Geometry: final body of the model. Coordinates: model frame, mm. Face numbers are marked on the shaded views. A direction names the side the tool comes from. Coordinates: 2 decimals unless noted, no trailing zeros. Loops run counter-clockwise (first coordinate to the right, second up) from the corner with the lowest first, then second, coordinate; pieces in that order, holes last. Notation, with made-up numbers: (42.5, -10.5) - (70.5, -10.5) arc R28 cw to (70.5, 9.5) - close; hole circle Ø6 at (-26, 83.25). An arc over 180 degrees is marked (long way). Put each result on its own line as item: value. Start each with the question number.
1) Section D-D on y = 1.5. Output: boundary loops of the cut face in (x, z).
2) Section B-B on z = -1.4. Output: boundary loops of the cut face in (x, y), and give its area (3 significant figures).
3) Section A-A on x = 2.75. Output: boundary loops of the cut face in (y, z).
4) Reachability of the marked faces 1, 2, 3 and 4 from +Z, -Z, +X, -X, +Y, -Y: full face, straight path, thin tool, end or side. Return the list, or none.
5) Section C-C on y = 17. Output: boundary loops of the cut face in (x, z).
6) Draft query along X for the marked faces 5, 6 and 7. Return one class per face: +X half, -X half, draft (parallel to the pull), parting line (faces both ways), or undercut.
7) Material intervals for line 1 along X through (y, z) = (15.5, -2.8); line 2 along X through (y, z) = (13.5, -1.95); line 3 along Y through (x, z) = (3.5, -2.05), sorted ascending. Write a range as from..to.
8) Contact query for a flat-ended pin moving along its axis: pin 1 Ø8 at (x, y) = (0.5, 5.5) entering from +Z. Output: stop coordinate, or through.
```python
from build123d import *

# Parameters (mm, degrees)
SKETCH_1_R      = 1.3
EXTRUDE_1_DEPTH = 3


with BuildPart() as part:
    # 草图1 → 凸台-拉伸1 (new body)
    with BuildSketch(Plane(origin=(0, 0, -3.362857667), x_dir=(-1, 0, 0), z_dir=(0, 0, -1))):
        with BuildLine():
            Line((-8.929456987, 17.45330102), (-12.208534908, 5.216337034))
            ThreePointArc((-12.208534908, 5.216337034), (-8.203956956, -0.691485495), (-5.819308033, 6.03550946))
            ThreePointArc((-5.819308033, 6.03550946), (-6.310108859, 6.921233679), (-6.304159928, 7.933833034))
            Line((-6.304159928, 7.933833034), (-4.539684391, 14.518557193))
            ThreePointArc((-4.539684391, 14.518557193), (-3.62301138, 15.532716808), (-2.264294404, 15.382060533))
            Line((-2.264294404, 15.382060533), (-0.142530428, 17.503217343))
            Line((-0.142530428, 17.503217343), (4.099819599, 13.25965297))
            Line((4.099819599, 13.25965297), (5.797509256, 14.956856814))
            Line((5.797509256, 14.956856814), (1.554532399, 19.201048196))
            Line((1.554532399, 19.201048196), (3.675778765, 21.321687543))
            Line((3.675778765, 21.321687543), (-4.808443123, 29.808337985))
            Line((-4.808443123, 29.808337985), (-6.931968366, 27.685420414))
            Line((-6.931968366, 27.685420414), (-11.173246227, 31.927912314))
            Line((-11.173246227, 31.927912314), (-12.870428791, 30.231215419))
            Line((-12.870428791, 30.231215419), (-8.629080401, 25.98865297))
            Line((-8.629080401, 25.98865297), (-10.749072595, 23.869267436))
            Line((-10.749072595, 23.869267436), (-10.611098311, 23.731253658))
            ThreePointArc((-10.611098311, 23.731253658), (-8.929299443, 20.817545637), (-8.929456987, 17.45330102))
        make_face()
        with Locations(Location((-3.536567574, 22.593983824, 0), (0, 0, 180))):
            Circle(SKETCH_1_R, mode=Mode.SUBTRACT)
        with Locations(Location((-8.71249984, 3.274951558, 0), (0, 0, 180))):
            Circle(SKETCH_1_R, mode=Mode.SUBTRACT)
    extrude(amount=-EXTRUDE_1_DEPTH)


solid = part.part
```
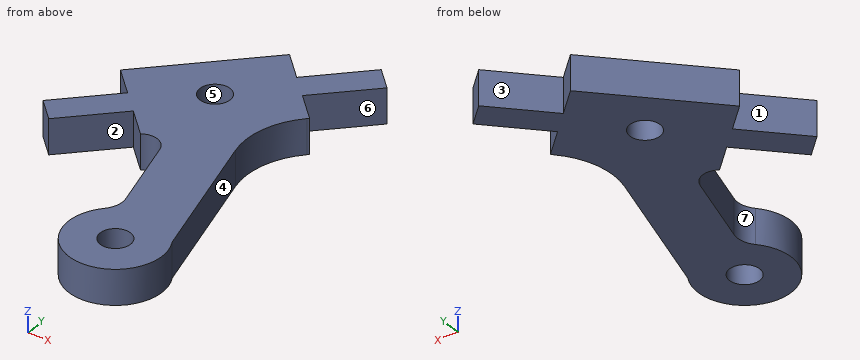
Answer block:
1. outline: (5.13, -3.36) - (12.3, -3.36) - (12.3, -0.36) - (5.13, -0.36) - close
2. outline: (-5.8, 14.96) - (-4.1, 13.26) - (0.14, 17.5) - (2.26, 15.38) arc R1.5 cw to (4.54, 14.52) - (6.3, 7.93) arc R2 cw to (5.82, 6.04) arc R4 ccw (long way) to (12.21, 5.22) - (8.93, 17.45) arc R6.5 cw to (10.61, 23.73) - (10.75, 23.87) - (8.63, 25.99) - (12.87, 30.23) - (11.17, 31.93) - (6.93, 27.69) - (4.81, 29.81) - (-3.68, 21.32) - (-1.55, 19.2) - close; hole circle Ø2.6 at (3.54, 22.59); hole circle Ø2.6 at (8.71, 3.27)
2. area: 236 mm²
3. outline: (15.59, -3.36) - (21.56, -3.36) - (21.56, -0.36) - (15.59, -0.36) - close; (23.63, -3.36) - (27.75, -3.36) - (27.75, -0.36) - (23.63, -0.36) - close
4. face 1: +Z, -Z, -X
4. face 2: +Z, -Z, -Y
4. face 3: +Z, -Z, +Y
4. face 4: +Z, -Z, +X
5. outline: (-3.75, -3.36) - (-0.36, -3.36) - (-0.36, -0.36) - (-3.75, -0.36) - close; (0.65, -3.36) - (9.05, -3.36) - (9.05, -0.36) - (0.65, -0.36) - close
6. face 5: undercut
6. face 6: +X half
6. face 7: -X half
7. line 1: x = -5.25..-1.86, 2.15..2.48, 3.7..9.45
7. line 2: x = -4.34..-3.86, 4.81..9.99
7. line 3: y = 15.57..21.29, 23.89..28.5
8. pin 1: passes through
